The model under review builds one solid part; all positions refer to its coordinate system, in mm. Round coordinates to 2 decimals unless told otherwise and drop trailing zeros. Order: outer loops, then holes, each group sorted by start corner. A loop starts at its lowest first (then second) coordinate and runs counter-clockwise, first axis right, second up. Notation, with made-up numbers: M 34,-9.75 L 54,-9.75 A21 ccw 54,20.25 Z; hole C -29,59 d10. An arc over 180 degrees is marked long. Answer as a JSON object with one key per item and string values. Group by question number.
1) Consider section C-C, the plane y = -153.5. Write out the cut boundary in (x, z), then the cut area to 3 significant figures.
2) To check wall thickness, follow line 1 (X direction, y = -534.5, z = -40); line 2 (Y direction, x = -124.5, z = -19); line 3 (Y direction, x = 173.5, z = -14.5). State the ranges of each line that lie inside material, in increasing order.
3) Consider section B-B, the plane x = 138. Write out the cut boundary in (y, z).
4) Consider section A-A, the plane z = -31. Write out the cut boundary in (x, y).
5) Insertion check: pin 1 Ø2 at (x, z) = (-77.5, -19.5) entering from +Y; pin 2 Ø1.5 at (y, z) = (-146.5, -6) entering from +X; pin 3 Ø10 at (x, z) = (111.5, -23) entering from -Y. Each pin has a flat end and moves straight along its axis. Give the tip position at first contact, or say it passes through.
Autodesk Inventor part; units mm, degrees
ref_plane "YZ Plane" through (0, 0, 0) normal (1, 0, 0) x (0, 1, 0)
ref_plane "XZ Plane" through (0, 0, 0) normal (0, 1, 0) x (-1, 0, 0)
ref_plane "XY Plane" through (0, 0, 0) normal (0, 0, 1) x (1, 0, 0)
ref_plane "Work Plane1" through (0, 0, 0) normal (0, 0, 1) x (1, 0, 0)
sketch "Sketch1" plane through (0, 0, 0) normal (0, 0, 1) x (1, 0, 0)
  line L0 (-190.5, -50.8) -> (190.5, -50.8)
  line L1 (-190.5, -609.6) -> (-190.5, -508)
  line L2 (190.5, -50.8) -> (-190.5, -609.6)
  line L3 (-190.5, -508) -> (-190.5, 1727.2)
  line L4 (-37.5923, -204.9815) -> (-190.5, -429.2461)
  line L5 (-37.5923, -204.9815) -> (67.5314, -50.8)
  line L6 (190.5, -50.8) -> (67.5314, -50.8)
  line L7 (-190.5, -429.2461) -> (-190.5, -609.6)
  point P0 (0, 0)
  point P1 (-190.5, -429.2461)
  dimension "d0" = 101.6
extrude "Extrusion1" add sketch "Sketch1" against normal blind 50.8 contours L0 L2 L1 L3 L4 L5
properties part number "Top of head diagonals"
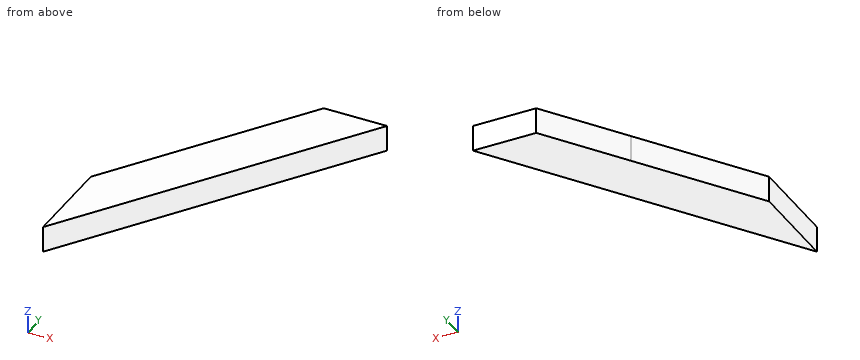
Results list:
{
 "1": {"outline": "M -2.49,-50.8 L 120.48,-50.8 L 120.48,0 L -2.49,0 Z", "area": "6,250 mm^2"},
 "2": {"line 1": "-190.5 to -139.3", "line 2": "-512.8 to -332.45", "line 3": "-75.73 to -50.8"},
 "3": {"outline": "M -127.8,-50.8 L -50.8,-50.8 L -50.8,0 L -127.8,0 Z"},
 "4": {"outline": "M -190.5,-609.6 L 190.5,-50.8 L 67.53,-50.8 L -37.59,-204.98 L -190.5,-429.25 Z"},
 "5": {"pin 1": "y = -262.05", "pin 2": "x = 125.76", "pin 3": "y = -174"}
}
